Source: three-view drawing plus pictorial views. Frame: mm from the lowest corner of the part. A direction names the side the tool comes from. Give positions to 0.01 mm unless a question says otherwise; leave off trailing zeros. Loops run counter-clockwise (first coordinate to the right, second up) from the corner with the lowest first, then second, coordinate; pieces in that order, holes last.
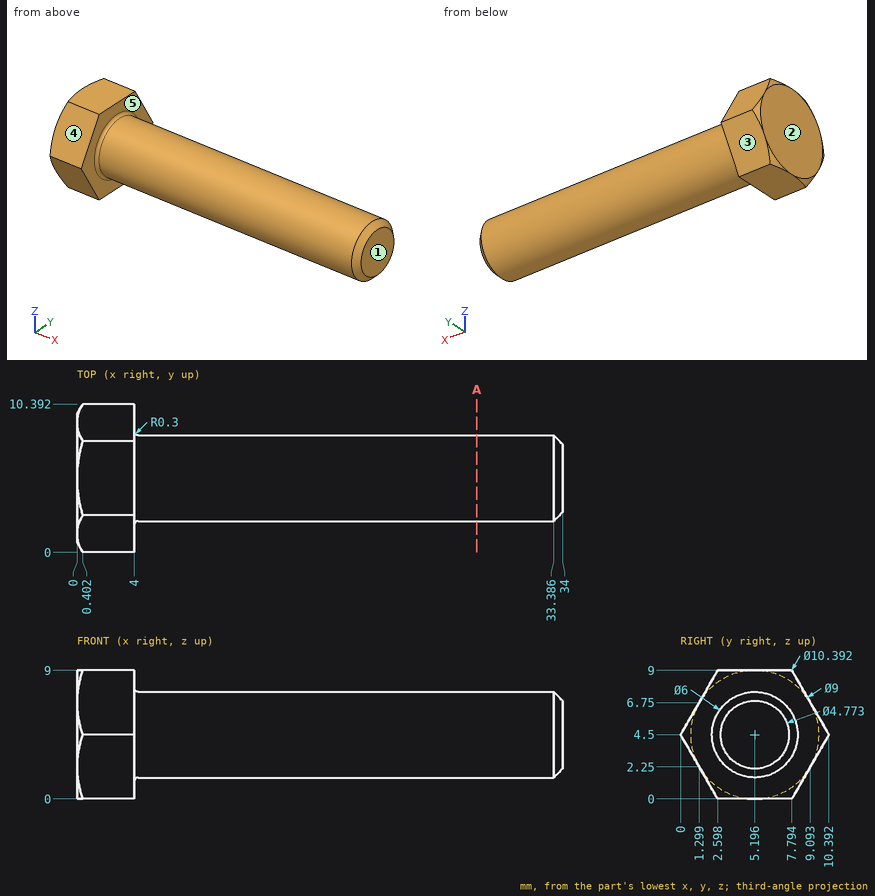
1) Contact query for flat-ended pins moving along their axis: P1, Ø1.5, axis at x = 5.5, y = 2.5, coming from the -Z side; P2, Ø4, axis at x = 26, z = 7, coming from the -Y side; P3, Ø6, axis at x = 28, y = 9, coming from the +Z side. Output: stop coordinate, or through.
Checks:
P1: stops at z = 2.22
P2: stops at y = 2.24
P3: stops at z = 7.39
2) Pull-direction query (X, two-part tool) for the marked faces 1, 2 and 3; classes: released by +X, released by -X, zero draft, split by the parting line, or undercut.
Checks:
face 1: released by +X
face 2: released by -X
face 3: zero draft
3) Reachability of the marked faces 4 and 5 from +Z, -Z, +X, -X, +Y, -Y: full face, straight path, thin tool, end or side. Return the list, or none.
Checks:
face 4: +Z, +X, -X, -Y
face 5: +X
4) Ray query, probe 1 along X at (y, z) = (7.5, 7.5); probe 2 along Y at (x, z) = (29, 6) (1 decimal); probe 3 along X at (y, z) = (4.25, 7) (1 decimal). Return the intervals inside material, ascending.
Checks:
probe 1: x = 0 to 4
probe 2: y = 2.6 to 7.8
probe 3: x = 0 to 33.7
5) Cut plane A-A (x = 28). Return loops of the section in (y, z), and give its area (3 significant figures).
Checks:
outline: circle Ø6 at (5.2, 4.5)
area: 28.3 mm2
